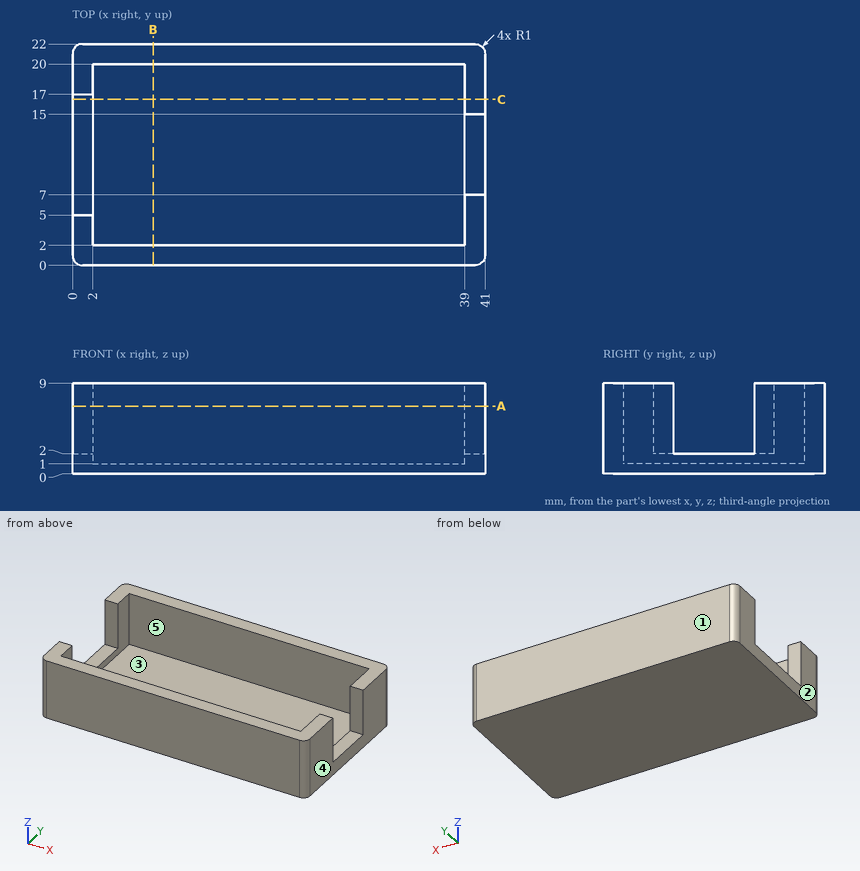
Part print with two shaded views. Sizes in mm from the minimum x, y, z corner. A direction names the side the tool comes from. Coordinates: 2 decimals unless noted, no trailing zeros. Write each loop counter-clockwise with the first axis right and the second up, starting at its lowest first coordinate (ties: lowest second). Pieces come first, ordered by that corner, then holes. Notation, with made-up numbers: M 21.25,46 L 39.25,46 A24 cw 39.25,69 Z; hole C 0,-37.5 d8. An arc over 180 degrees is marked long. Return JSON: item names as keys, results as strings.
Item 1: Which spindle directions (+Z, -Z, +X, -X, +Y, -Y) get a long thin tool onto all of the face, cutting with end or side? Do the marked faces 4 and 5. Say none if no direction does.
Findings below:
{"face 4": "+Z, -Z, +X, +Y, -Y", "face 5": "+Z"}
Item 2: Slice it at B-B, the plane x = 8. Write the cut outline in (y, z).
Findings below:
{"outline": "M 0,0 L 22,0 L 22,9 L 20,9 L 20,1 L 2,1 L 2,9 L 0,9 Z"}
Item 3: Slice it at A-A, the plane z = 6.75. Write the cut outline in (x, y).
Findings below:
{"outline": "M 0,1 A1 ccw 1,0 L 40,0 A1 ccw 41,1 L 41,7 L 39,7 L 39,2 L 2,2 L 2,5 L 0,5 Z; M 0,17 L 2,17 L 2,20 L 39,20 L 39,15 L 41,15 L 41,21 A1 ccw 40,22 L 1,22 A1 ccw 0,21 Z"}
Item 4: Drop flat-ended pins along their axis: pin 1 Ø2 at (x, z) = (36, 3.5) entering from -Y; pin 2 Ø2 at (x, y) = (1, 10.5) entering from +Z; pin 3 Ø3 at (y, z) = (14, 5) entering from -X; pin 4 Ø9 at (x, y) = (26, 9.5) entering from +Z. Give the stop position or say it passes through.
Findings below:
{"pin 1": "stops at y = 0", "pin 2": "stops at z = 2", "pin 3": "stops at x = 39", "pin 4": "stops at z = 1"}
Item 5: Two-plate mould, pull along X, no slides. Class the marked faces 1, 2 and 3: +X half, -X half, draft (parallel to the pull), parting line (faces both ways), or undercut.
Findings below:
{"face 1": "draft", "face 2": "-X half", "face 3": "undercut"}
Item 6: Slice it at C-C, the plane y = 16.5. Write the cut outline in (x, z).
Findings below:
{"outline": "M 0,0 L 41,0 L 41,9 L 39,9 L 39,1 L 2,1 L 2,2 L 0,2 Z"}
Item 7: Probe line 1 (Y direction, x = 11, z = 2.25); line 2 (X direction, y = 4.75, z = 2.5); line 3 (Y direction, x = 39.5, z = 7). List the from-to ranges inside material, lowest first. Write a range as from..to.
Findings below:
{"line 1": "y = 0..2, 20..22", "line 2": "x = 0..2, 39..41", "line 3": "y = 0..7, 15..22"}
